from build123d import *

# Parameters (mm, degrees)
F1_DEPTH = 10


# Not quite as in the source:
# - a feature of the source that left no trace in its solid (it failed there, or was rolled back) is left out


with BuildPart() as f1:
    # F0 (on Top) → F1 (new body)
    with BuildSketch(Plane.XY):
        with BuildLine():
            Line((-29.9939722279, 12.9722623931), (-42.3191245349, 25.9821456543))
            Line((-42.3191245349, 25.9821456543), (-49.6405097403, 1.341635914))
            Line((-49.6405097403, 1.341635914), (-29.3788570259, 6.1880200524))
            ThreePointArc((-29.3788570259, 6.1880200524), (-14.4470126823, -3.3975764275), (-23.2838200208, -18.7844042826))
            ThreePointArc((-23.2838200208, -18.7844042826), (-23.9549101464, -18.9642061938), (-24.6347260756, -19.1075274636))
            Line((-24.6347260756, -19.1075274636), (-43.6607604489, -23.658364086))
            Line((-43.6607604489, -23.658364086), (-25.9821456543, -42.3191245349))
            Line((-25.9821456543, -42.3191245349), (-20.4059776484, -23.5522357279))
            ThreePointArc((-20.4059776484, -23.5522357279), (-20.2283734176, -22.8904168158), (-20.0157770781, -22.2389950387))
            ThreePointArc((-20.0157770781, -22.2389950387), (-4.0233304879, -14.28870031), (4.4989162669, -29.9838219872))
            ThreePointArc((4.4989162669, -29.9838219872), (4.4318374321, -30.2176557723), (4.3603484872, -30.4501791902))
            Line((4.3603484872, -30.4501791902), (-1.341635914, -49.6405097403))
            Line((-1.341635914, -49.6405097403), (23.658364086, -43.6607604489))
            Line((23.658364086, -43.6607604489), (10.2042067758, -29.4591496596))
            ThreePointArc((10.2042067758, -29.4591496596), (9.7129486903, -28.9678695182), (9.2489208652, -28.4507922885))
            ThreePointArc((9.2489208652, -28.4507922885), (10.2477999291, -10.735096536), (27.9912063973, -10.8582317502))
            Line((27.9912063973, -10.8582317502), (42.3191245349, -25.9821456543))
            Line((42.3191245349, -25.9821456543), (49.6405097403, -1.341635914))
            Line((49.6405097403, -1.341635914), (32.2110441824, -5.5105892868))
            ThreePointArc((32.2110441824, -5.5105892868), (30.1080602508, -6.2077620929), (27.9172204019, -6.5376288751))
            ThreePointArc((27.9172204019, -6.5376288751), (14.3772643763, 3.7032958994), (22.517444526, 18.6010949497))
            ThreePointArc((22.517444526, 18.6010949497), (24.0610630231, 19.0733865517), (25.6513214754, 19.3506868884))
            Line((25.6513214754, 19.3506868884), (43.6607604489, 23.658364086))
            Line((43.6607604489, 23.658364086), (25.9821456543, 42.3191245349))
            Line((25.9821456543, 42.3191245349), (20.7505372467, 24.7118693081))
            ThreePointArc((20.7505372467, 24.7118693081), (20.3589951368, 22.9556577497), (19.7280350427, 21.2705839763))
            ThreePointArc((19.7280350427, 21.2705839763), (4.1315999448, 14.2550710192), (-4.8477844397, 28.8096876713))
            ThreePointArc((-4.8477844397, 28.8096876713), (-4.4924498123, 30.3397177103), (-3.9546627515, 31.8155360239))
            Line((-3.9546627515, 31.8155360239), (1.341635914, 49.6405097403))
            Line((1.341635914, 49.6405097403), (-23.658364086, 43.6607604489))
            Line((-23.658364086, 43.6607604489), (-10.9230867149, 30.2179673888))
            ThreePointArc((-10.9230867149, 30.2179673888), (-9.7422609409, 29.1173003575), (-8.7069825787, 27.8787463076))
            ThreePointArc((-8.7069825787, 27.8787463076), (-10.0224304809, 10.9531282619), (-26.9576179635, 9.767221714))
            ThreePointArc((-26.9576179635, 9.767221714), (-28.6128792901, 11.2398728194), (-29.9939722279, 12.9722623931))
        make_face()
    extrude(amount=F1_DEPTH)


solid = f1.part
The listing builds one solid part. Answer for the finished solid, in the listing's coordinates (mm). A direction names the side the tool comes from. Round coordinates to 2 decimals unless told otherwise and drop trailing zeros. Write each loop counter-clockwise with the first axis right and the second up, starting at its lowest first coordinate (ties: lowest second). Pieces come first, ordered by that corner, then holes. Notation, with made-up numbers: M -9,-13.75 L 4,-13.75 A17 cw 4,17.25 Z; hole C 32.5,55 d6. An arc over 180 degrees is marked long. Write each question's results on one line, items separated by ' | '. Start each with the question number.
Item 1: For a pull along X with two mould halves and no side action, classify faces 1 (the face through (-36.07, 19.386, 4.93)), 2 (the face through (10.983, -46.692, 4.93)), 3 (the face through (-1.344, 40.603, 4.93)), 4 (the face through (-17.38, 37.033, 4.93)) as pulls with the +X half, pulls with the -X half, needs draft (parallel to the pull), parting line crosses it, or undercut.
Item 2: A cutting plane is placed at C-C on z = 6.25. Write down the section's boundary in (x, y), and give its area (3 significant figures).
Item 3: For faces 5 (the face through (-23.233, -33.067, 4.93)), 6 (the face through (17.025, -36.659, 4.93)), 7 (the face through (41.048, -3.397, 4.93)), determine the directions among +Z, -Z, +X, -X, +Y, -Y from which every point of the face is accessible in a straight line to the end or side of a thin tool.
Item 4: Straight lines are drawn through the part: L1, parallel to Y at x = 18.5, z = 3.5; L2, parallel to Y at x = 17, z = 8.25; L3, parallel to Y at x = 8, z = 7.5. For each, find the intervals that lie inside material, in ascending order. Write a range as [from, to].
Item 5: Flat-ended cylindrical pins translate along their axes: pin 1 Ø2 at (y, z) = (28, 1) entering from +X (3 decimals); pin 2 Ø3 at (x, z) = (35, 5) entering from -Y; pin 3 Ø4 at (y, z) = (29, 3.5) entering from -X; pin 4 Ø12 at (x, y) = (10.5, 21.5) entering from +Z. Find the tip coordinate at first contact, or state that the pin passes through.
Item 6: A cutting plane is placed at D-D on y = 4. Write down the section's boundary in (x, z), and give its area (3 significant figures).
Item 7: A cutting plane is placed at A-A on y = -36.5. Write down the section's boundary in (x, z) (3 decimals).
Item 8: A cutting plane is placed at B-B on y = -21. Write down the section's boundary in (x, z), and give its area (3 significant figures).
Check sheet entries:
1) face 1: undercut | face 2: pulls with the +X half | face 3: undercut | face 4: pulls with the -X half
2) outline: M -49.64,1.34 L -29.38,6.19 A12.87 cw long -24.63,-19.11 L -43.66,-23.66 L -25.98,-42.32 L -20.41,-23.55 A12.86 cw long 4.36,-30.45 L -1.34,-49.64 L 23.66,-43.66 L 10.2,-29.46 A12.87 cw long 27.99,-10.86 L 42.32,-25.98 L 49.64,-1.34 L 32.21,-5.51 A13 cw long 25.65,19.35 L 43.66,23.66 L 25.98,42.32 L 20.75,24.71 A12.96 cw long -3.95,31.82 L 1.34,49.64 L -23.66,43.66 L -10.92,30.22 A13 cw long -29.99,12.97 L -42.32,25.98 Z | area: 2,710 mm²
3) face 5: +Z, -Z, -Y | face 6: +Z, -Z, +X | face 7: +Z, -Z
4) L1: [-44.89, -38.22], [-7.26, -3.33], [16.19, 19.14] | L2: [-45.25, -36.63], [-7.41, -1.77], [14.63, 17.38] | L3: [-47.41, -26.7], [-13.53, 13.69]
5) pin 1: x = 40.495 | pin 2: y = -19.84 | pin 3: x = -11.66 | pin 4: through
6) outline: M -48.85,0 L -38.53,0 L -38.53,10 L -48.85,10 Z; M -19.44,0 L 14.32,0 L 14.32,10 L -19.44,10 Z | area: 441 mm²
7) outline: M -31.495,0 L -24.253,0 L -24.253,10 L -31.495,10 Z; M 2.563,0 L 16.874,0 L 16.874,10 L 2.563,10 Z
8) outline: M -32.55,0 L -19.5,0 L -19.5,10 L -32.55,10 Z; M 3.7,0 L 6.22,0 L 6.22,10 L 3.7,10 Z; M 37.6,0 L 43.8,0 L 43.8,10 L 37.6,10 Z | area: 218 mm²
